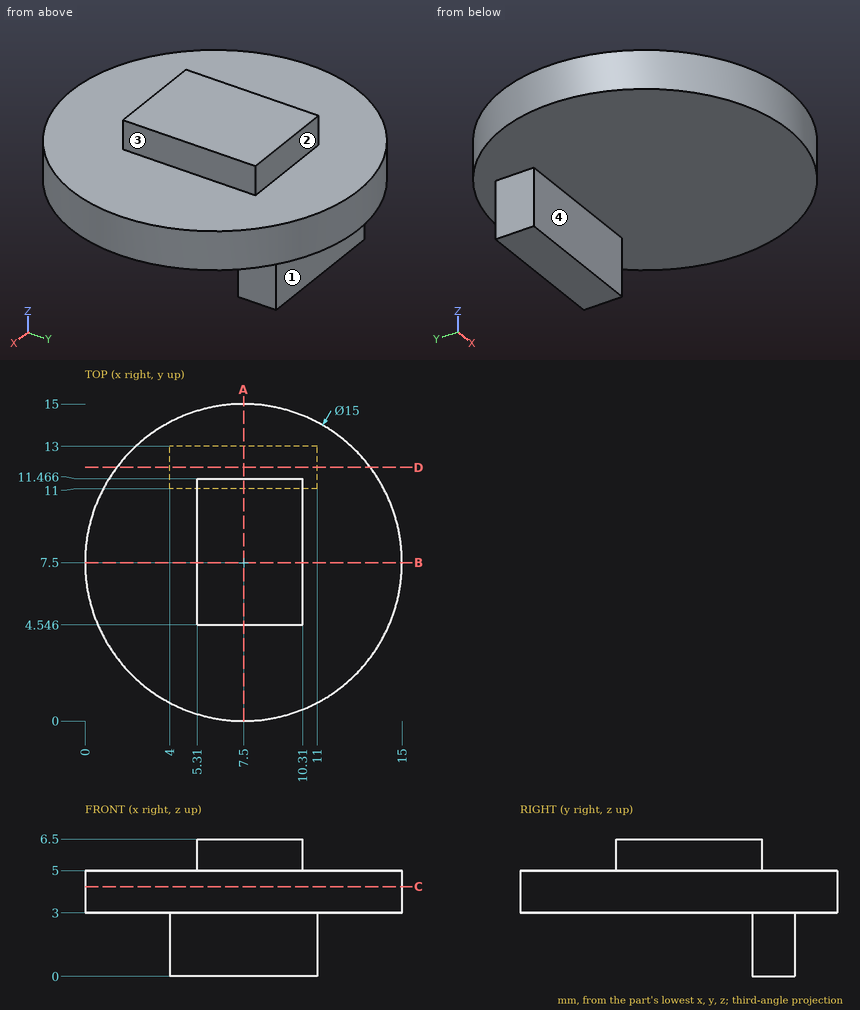
Answer from the drawing. Dimensions are ordinates in mm from the lowest x, y and z of the part. A direction names the side the tool comes from. Round coordinates to 2 decimals unless told otherwise and drop trailing zeros. Order: outer loops, then holes, each group sorted by start corner. A loop starts at its lowest first (then second) coordinate and runs counter-clockwise, first axis right, second up. Notation, with made-up numbers: (-27.5, 28.25) - (20.5, 28.25) arc R21 cw to (20.5, 34.25) - close; hole circle Ø4 at (-6.5, 4). An arc over 180 degrees is marked (long way). Put each result on its own line as item: value. Start each with the question number.
(1) Straight lines are drawn through the part: probe 1 along X at (y, z) = (11.25, 1.5); probe 2 along Y at (x, z) = (4.25, 0.5); probe 3 along Z at (x, y) = (9.5, 12). For each, find the intervals that lie inside material, in ascending order. Write a range as from..to.
(2) Given P1, Ø7.5, axis at x = 9.5, y = 8.5, coming from the -Z side; P2, Ø1, axis at x = 10, y = 7, coming from the -Z side; P3, Ø1.6, axis at y = 8.5, z = 5.5, coming from the -X side; P4, Ø3, axis at x = 5, z = 3, coming from the +Y side, each flat-ended and moving along its own axis, determine where each tip first touches the part or whether it passes through.
(3) Find section B-B (y = 7.5). Give the vertices of the cut face in (x, z), plus the area to 3 significant figures.
(4) For the marked faces 1, 2, 3 and 4, determine the directions among +Z, -Z, +X, -X, +Y, -Y from which every point of the face is accessible in a straight line to the end or side of a thin tool.
(5) Find section D-D (y = 12). Give the vertices of the cut face in (x, z).
(6) Find section C-C (z = 4.25). Give the vertices of the cut face in (x, y).
(7) Find section A-A (x = 7.5). Give the vertices of the cut face in (y, z) (1 decimal).
Reply:
1. probe 1: 4..11
1. probe 2: 11..13
1. probe 3: 0..5
2. P1: z = 0
2. P2: z = 3
2. P3: x = 0.01
2. P4: y = 14.93
3. outline: (0, 3) - (15, 3) - (15, 5) - (10.31, 5) - (10.31, 6.5) - (5.31, 6.5) - (5.31, 5) - (0, 5) - close
3. area: 37.5 mm^2
4. face 1: -Z, +X, -X, +Y
4. face 2: +Z, +X, -X, +Y
4. face 3: +Z, +X, +Y, -Y
4. face 4: -Z, +X, -X, -Y
5. outline: (1.5, 3) - (4, 3) - (4, 0) - (11, 0) - (11, 3) - (13.5, 3) - (13.5, 5) - (1.5, 5) - close
6. outline: circle Ø15 at (7.5, 7.5)
7. outline: (0, 3) - (11, 3) - (11, 0) - (13, 0) - (13, 3) - (15, 3) - (15, 5) - (11.5, 5) - (11.5, 6.5) - (4.5, 6.5) - (4.5, 5) - (0, 5) - close
